Input: part model. Units: mm. Frame: model coordinates. A direction names the side the tool comes from. Coordinates: 2 decimals unless noted, no trailing zeros. Write each loop counter-clockwise with the first axis right and the second up, starting at its lowest first coordinate (ties: lowest second). Pieces come first, ordered by that corner, then holes. Notation, with made-up numbers: (-2, -14) - (14, -14) arc R17 cw to (14, 2) - close; hole circle Ø7 at (51.25, 76). An arc over 180 degrees is marked (long way). Use a Markdown table: item, result. Add a question column.
Q1. Section query A-A (z = -8). Return the cut outline in (x, y) (3 decimals).
Q2. Pin query (flat end, axial travel): P1, Ø6, axis at y = 21.5, z = -14.5, coming from the +X side; P2, Ø2.5, axis at y = 22, z = -8.5, coming from the -X side; P3, Ø3, axis at x = -1.5, z = 12.5, coming from the -Y side; P4, Ø5, axis at x = 19.5, y = 25, coming from the -Z side. Return the tip coordinate at first contact, or that it passes through.
Q3. Section query D-D (x = -15). Return the cut outline in (y, z).
Q4. Section query C-C (z = 0). Return the cut outline in (x, y) (3 decimals).
Q5. Set-up query: faces 1 (the face through (0, -3, 25.4)), 2 (the face through (0.879, 9.543, 22.328)), 3 (the face through (4.2, 22.56, 4.24)), 4 (the face through (0, 16.248, 14)). Return all of +Z, -Z, +X, -X, +Y, -Y with unobstructed straight access to the full face (end or side cutting, diameter ignored); none if empty.
Q6. Material intervals for probe 1 along Z at (x, y) = (0, 20) (3 decimals); probe 2 along Z at (x, y) = (-11, 22); probe 3 along Y at (x, z) = (-4, -13), sorted ascending. Write a range as from..to.
Q7. Mould query, pull axis X, two halves, no side actions, for faces 5 (the face through (-1, -3, 22.86)), 6 (the face through (-4.2, 22.56, -4.24)), 7 (the face through (0, 20.955, 1)), 8 (the face through (-1.27, -7, 24)). Classes: released by +X, released by -X, zero draft, split by the parting line, or undercut.
Autodesk Inventor part; units mm, degrees
ref_plane "Work Plane1" through (0, 6.35, 25.4) normal (0, 0, 1) x (1, 0, 0)
ref_plane "Work Plane2" through (0, 24.13, 0) normal (0, 1, 0) x (1, 0, 0)
ref_plane "Work Plane4" through (0, 20.955, 12.4434) normal (1, 0, 0) x (0, 0, -1)
sketch "Sketch1" plane through (0, 0, 0) normal (0, 1, 0) x (-1, 0, 0)
  circle A0 centre (0, 0) radius 25.4
  dimension "d0" = 50.8
extrude "Extrusion1" add sketch "Sketch1" along normal blind 6.35
sketch "Sketch2" plane through (0, 6.35, 0) normal (0, 1, 0) x (1, 0, 0)
  circle A0 centre (0, 0) radius 25.4
  point P0 (-25.4, 0)
  point P1 (0, -25.4)
  point P2 (25.4, 0)
  point P3 (0, 25.4)
ref_plane "Work Plane1" through (0, 6.35, 25.4) normal (0, 0, 1) x (1, 0, 0)
sketch "Sketch3" plane through (0, 6.35, 25.4) normal (0, 0, 1) x (1, 0, 0)
  line L0 (1.27, -4.1248) -> (-1.27, -4.1248)
  line L1 (-1.27, -4.1248) -> (-1.27, -14.6393)
  line L2 (-1.27, -14.6393) -> (1.27, -14.6393)
  line L3 (1.27, -14.6393) -> (1.27, -4.1248)
  line L4 (25.4, 0) -> (-25.4, 0)
  line L5 (0, 0) -> (0, -6.35)
  dimension "d3" = 1.27
  dimension "d4" = 2.54
extrude "Extrusion2" add sketch "Sketch3" against normal blind 2.54
sketch "Sketch4" plane through (0, 6.35, 0) normal (0, 1, 0) x (1, 0, 0)
  circle A0 centre (0, 0) radius 6.4452
  dimension "d9" = 12.8905
extrude "Extrusion3" cut sketch "Sketch4" against normal blind 25.4
sketch "Sketch5" plane through (0, 6.35, 0) normal (0, 1, 0) x (1, 0, 0)
  circle A0 centre (0, 0) radius 15.875
  dimension "d12" = 31.75
extrude "Extrusion4" add sketch "Sketch5" along normal blind 22.86
sketch "Sketch6" plane through (0, 29.21, 0) normal (0, 1, 0) x (1, 0, 0)
  circle A0 centre (0, 0) radius 12.7
  dimension "d15" = 25.4
extrude "Extrusion5" cut sketch "Sketch6" against normal blind 19.05
sketch "Sketch7" plane through (0, 0, 0) normal (0, -1, 0) x (1, 0, 0)
  point P0 (0, 0)
sketch "Sketch8" plane through (0, 0, 0) normal (0, -1, 0) x (1, 0, 0)
  point P0 (0, 0)
sketch "Sketch9" plane through (0, 0, 0) normal (0, -1, 0) x (1, 0, 0)
  point P0 (0, 0)
sketch "Sketch10" plane through (0, 0, 0) normal (0, -1, 0) x (1, 0, 0)
  point P0 (0, 0)
ref_plane "Work Plane2" through (0, 24.13, 0) normal (0, 1, 0) x (1, 0, 0)
sketch "Sketch13" plane through (0, 24.13, 0) normal (0, 1, 0) x (1, 0, 0)
  circle A0 centre (0, 0) radius 12.7
  circle A1 centre (0, 0) radius 12.7
  circle A2 centre (0, 0) radius 5.969
  line L0 (0, 12.7) -> (2.54, 12.7)
  line L1 (0, 12.7) -> (-2.54, 12.7)
  line L2 (0, -12.7) -> (2.54, -12.7)
  line L3 (2.54, -12.7) -> (2.54, 12.7)
  line L4 (0, -12.7) -> (-2.54, -12.7)
  line L5 (-2.54, -12.7) -> (-2.54, 12.7)
  line L6 (12.7, -2.54) -> (-12.7, -2.54)
  line L7 (-12.7, 0) -> (-12.7, -2.54)
  line L8 (-12.7, 0) -> (-12.7, 2.54)
  line L9 (12.7, 2.54) -> (-12.7, 2.54)
  line L10 (12.7, 0) -> (12.7, 2.54)
  line L11 (12.7, 0) -> (12.7, -2.54)
  point P0 (12.4434, -2.54)
  point P1 (5.4016, -2.54)
  point P2 (2.54, -5.4016)
  point P3 (2.54, -12.4434)
  point P4 (-5.4016, -2.54)
  point P5 (-12.4434, -2.54)
  point P6 (-2.54, -12.4434)
  point P7 (-2.54, -5.4016)
  point P8 (5.4016, 2.54)
  point P9 (12.4434, 2.54)
  point P10 (2.54, 12.4434)
  point P11 (2.54, 5.4016)
  point P12 (-12.4434, 2.54)
  point P13 (-5.4016, 2.54)
  point P14 (-2.54, 5.4016)
  point P15 (-2.54, 12.4434)
  dimension "d22" = 11.938
  dimension "d28" = 2.54
  dimension "d29" = 2.54
  dimension "d32" = 90
extrude "Extrusion6" add sketch "Sketch13" against normal blind 3.175 contours A0 L6 A2 L9 | L9 A2 L3 A0 | A0 L3 A2 L6 | L3 A2 L5 A0 | L9 L3 A2 | A2 L6 L3 L9 | A0 L5 A2 L3 | A2 L3 L6 | L3 L9 L5 A2 | L3 L6 L5 L9 | A2 L5 L6 L3 | L5 A2 L9 A0 | L5 L9 A2 | L5 L6 A2 L9 | A0 L6 A2 L5 | A2 L6 L5 | L9 A2 L6 A0
extrude "Extrusion7" cut sketch "Sketch13" against normal blind 3.175 contours L9 A2 L3 A0 | A0 L3 A2 L6 | L5 A2 L9 A0 | A0 L6 A2 L5
sketch "Sketch14" plane through (0, 6.35, 25.4) normal (0, 0, 1) x (1, 0, 0)
  line L0 (-12.7, 3.81) -> (12.7, 3.81)
  line L1 (-7.62, 9.8976) -> (7.62, 9.8976)
  line L2 (7.62, 9.8976) -> (7.62, 3.81)
  line L3 (7.62, 3.81) -> (-7.62, 3.81)
  line L4 (-7.62, 3.81) -> (-7.62, 9.8976)
  point P0 (0, -6.35)
  point P1 (-7.62, 3.81)
  dimension "d36" = 15.24
  dimension "d37" = 7.62
extrude "Extrusion8" cut sketch "Sketch14" against normal through all
sketch "Sketch15" plane through (0, 6.35, 0) normal (0, 1, 0) x (1, 0, 0)
  circle A0 centre (0, -20.6375) radius 1.905
  circle A1 centre (0, 0) radius 15.875
  circle A2 centre (0, 0) radius 25.4
  dimension "d40" = 3.81
ref_plane "Work Plane4" through (0, 20.955, 12.4434) normal (1, 0, 0) x (0, 0, -1)
sketch "Sketch17" plane through (0, 20.955, 12.4434) normal (1, 0, 0) x (0, 0, -1)
  line L0 (-6.2891, -14.605) -> (-10.0991, -14.605)
  line L1 (-8.1941, -14.605) -> (-8.1941, -10.16)
  line L2 (-11.3691, -6.985) -> (-12.9566, -6.985)
  arc A0 (-8.1941, -10.16) -> (-11.3691, -6.985) centre (-11.3691, -10.16) ccw
  point P0 (12.4434, -20.955)
  point P1 (-8.1941, -6.985)
  dimension "d46" = 7.62
  dimension "d47" = 4.7625
  dimension "d48" = 3.175
sweep "Sweep1" add profiles "Sketch15" path "Sketch17" path curves L1 A0 L2 contours A0
fillet "Fillet1" radius 1.905 1 edges at (-1.905, 13.97, 25.4)
fillet "Fillet2" radius 1.905 1 edges at (-1.905, 6.35, 20.6375)
fillet "Fillet3" radius 6.35 1 edges at (-1.27, 0, 24.1141)
properties part number "Wheel"
Values follow:
| question | item | result |
|---|---|---|
| 1 | outline | (-24.107, 0) - (24.107, 0) - (24.107, 6.35) - (13.712, 6.35) - (13.712, 29.21) - (9.864, 29.21) - (9.864, 10.16) - (-9.864, 10.16) - (-9.864, 29.21) - (-13.712, 29.21) - (-13.712, 6.35) - (-24.107, 6.35) - close; (-2.54, 20.955) - (2.54, 20.955) - (2.54, 24.13) - (-2.54, 24.13) - close |
| 2 | P1 | x = 10.94 |
| 2 | P2 | x = -14.12 |
| 2 | P3 | y = 0 |
| 2 | P4 | through |
| 3 | outline | (0, -20.5) - (6.35, -20.5) - (6.35, -5.2) - (29.21, -5.2) - (29.21, 5.2) - (6.35, 5.2) - (6.35, 20.5) - (0, 20.5) - close |
| 4 | outline | (-25.4, 0) - (-6.445, 0) - (-6.445, 6.35) - (6.445, 6.35) - (6.445, 0) - (25.4, 0) - (25.4, 6.35) - (15.875, 6.35) - (15.875, 29.21) - (12.7, 29.21) - (12.7, 24.13) - (-12.7, 24.13) - (-12.7, 29.21) - (-15.875, 29.21) - (-15.875, 6.35) - (-25.4, 6.35) - close; hole (-12.7, 10.16) - (12.7, 10.16) - (12.7, 20.955) - (-12.7, 20.955) - close |
| 5 | face 1 | +Z, +X, -X, +Y, -Y |
| 5 | face 2 | none |
| 5 | face 3 | +Y |
| 5 | face 4 | +Z, -Z |
| 6 | probe 1 | -15.875..-12.7, 12.7..15.875 |
| 6 | probe 2 | -11.45..-6.35, -2.54..2.54, 6.35..11.45 |
| 6 | probe 3 | 0..10.16, 16.25..29.21 |
| 7 | face 5 | zero draft |
| 7 | face 6 | undercut |
| 7 | face 7 | undercut |
| 7 | face 8 | released by -X |
